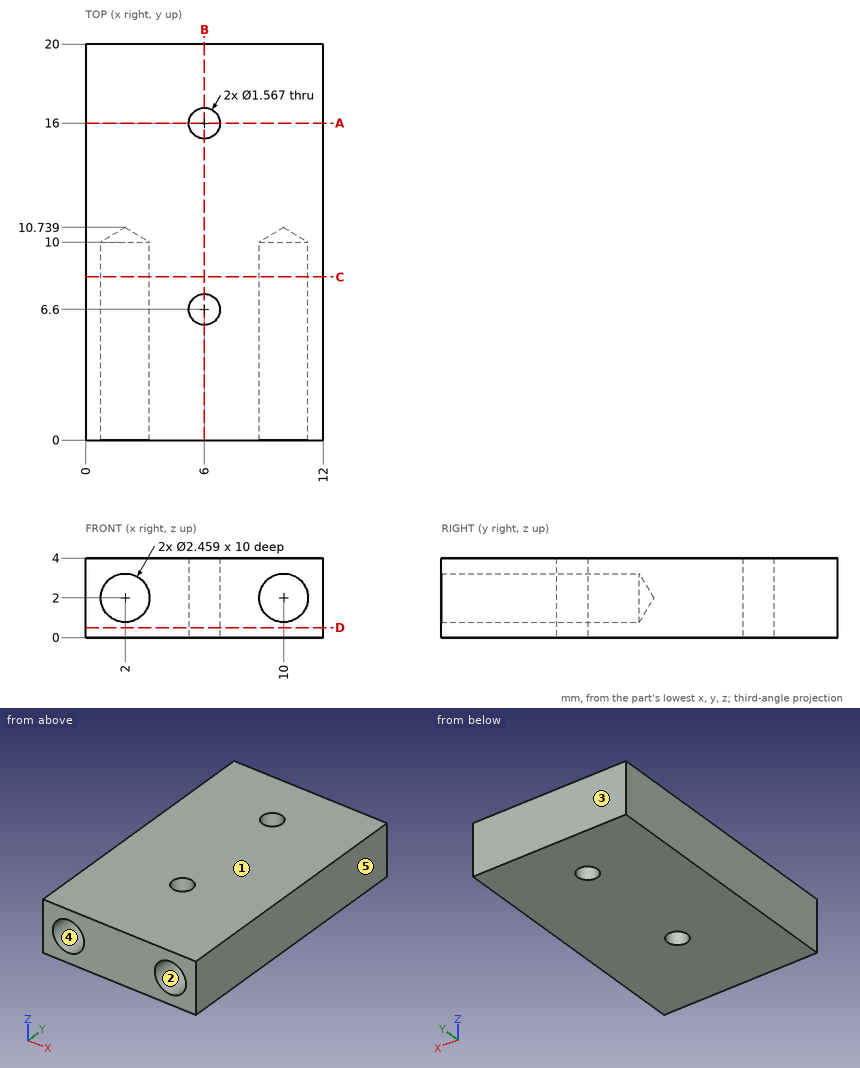
Answer from the drawing. Dimensions are ordinates in mm from the lowest x, y and z of the part. A direction names the side the tool comes from. Coordinates: 2 decimals unless noted, no trailing zeros. Order: outer loops, then holes, each group sorted by start corner. A loop starts at its lowest first (then second) coordinate and runs counter-clockwise, first axis right, second up. Notation, with made-up numbers: (-1, 45) -> (20, 45) arc R22 cw to (20, 77) -> close; hole circle Ø10 at (17.5, 71.25). An arc over 180 degrees is marked (long way). Answer as a JSON object with one key per item and string values.
1) Consider line 1 along Y through (x, z) = (6, 1.8); line 2 along X through (y, z) = (6.6, 1.9) (1 decimal); line 3 along X through (y, z) = (3.75, 2). Determine where each line is inside the solid, lowest interval first. Write a range as from..to.
Model answer:
{"line 1": "y = 0..5.82, 7.38..15.22, 16.78..20", "line 2": "x = 0..0.8, 3.2..5.2, 6.8..8.8, 11.2..12", "line 3": "x = 0..0.77, 3.23..8.77, 11.23..12"}
2) A cutting plane is placed at C-C, the plane y = 8.25. Determine the outline of the cut face in (x, z).
Model answer:
{"outline": "(0, 0) -> (12, 0) -> (12, 4) -> (0, 4) -> close; hole circle Ø2.46 at (2, 2); hole circle Ø2.46 at (10, 2)"}
3) A cutting plane is placed at D-D, the plane z = 0.5. Determine the outline of the cut face in (x, y), plus the area to 3 significant figures.
Model answer:
{"outline": "(0, 0) -> (12, 0) -> (12, 20) -> (0, 20) -> close; hole circle Ø1.57 at (6, 6.6); hole circle Ø1.57 at (6, 16)", "area": "236 mm²"}
4) The mould has two halves that part along X. Classify the marked faces 3, 4 and 5: released by +X, released by -X, zero draft, split by the parting line, or undercut.
Model answer:
{"face 3": "zero draft", "face 4": "undercut", "face 5": "released by +X"}
5) A cutting plane is placed at B-B, the plane x = 6. Determine the outline of the cut face in (y, z).
Model answer:
{"outline": "(0, 0) -> (5.82, 0) -> (5.82, 4) -> (0, 4) -> close; (7.38, 0) -> (15.22, 0) -> (15.22, 4) -> (7.38, 4) -> close; (16.78, 0) -> (20, 0) -> (20, 4) -> (16.78, 4) -> close"}
6) A cutting plane is placed at A-A, the plane y = 16. Determine the outline of the cut face in (x, z).
Model answer:
{"outline": "(0, 0) -> (5.22, 0) -> (5.22, 4) -> (0, 4) -> close; (6.78, 0) -> (12, 0) -> (12, 4) -> (6.78, 4) -> close"}
7) This flat-tipped pin is pushed along its axis until it touches: pin 1 (0.9 mm diameter, centred on x = 6, y = 16, fed in from +Z). Where does it stop, or does it pass through?
Model answer:
{"pin 1": "passes through"}
8) A tool of negligible diameter and unlimited length cuts with its end or side. For the marked faces 1 and 2, from which of +Z, -Z, +X, -X, +Y, -Y can it reach the whole face along a straight path? Write none if from no direction.
Model answer:
{"face 1": "+Z, +X, -X, +Y, -Y", "face 2": "-Y"}
